Read the model definition and answer for the solid it produces. Units are mm, in the model's axes. Coordinates: 2 decimals unless noted, no trailing zeros. Order: outer loops, then holes, each group sorted by start corner. A loop starts at its lowest first (then second) coordinate and runs counter-clockwise, first axis right, second up. Notation, with made-up numbers: (61, 0.5) -> (67, 0.5) arc R25 ccw to (67, 24.5) -> close; hole circle Ø1 at (-13, 55). An arc over 180 degrees is marked (long way). Use CSV: the item, a comma, the result in double quotes.
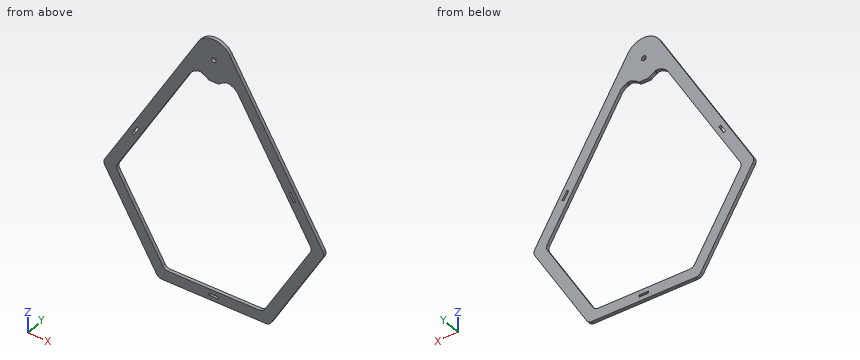
```python
from build123d import *

# Parameters (mm, degrees)
SKETCH1_R           = 4
BOSS_EXTRUDE1_DEPTH = 5.63
FILLET1_R           = 10
FILLET2_R           = 30
FILLET4_R           = 5


with BuildPart() as part:
    # Sketch1 → Boss-Extrude1 (new body)
    with BuildSketch(Plane(origin=(0, 0, 0), x_dir=(1, 0, 0), z_dir=(0, 1, 0))):
        Polygon((-36.68543943, -242.805029456), (146.099170261, 73.78720137), (54.706865415, 232.083316783), (-128.077744275, 232.083316783), (-219.470049121, 73.78720137), align=None)
        with Locations(Location((-36.68543943, -177.805029456, 0), (0, 0, 270))):
            Circle(SKETCH1_R, mode=Mode.SUBTRACT)
        with BuildLine():
            Line((67.466052068, -26.409354497), (3.019043242, -138.03484818))
            ThreePointArc((3.019043242, -138.03484818), (-2.040687786, -143.738783032), (-8.93543943, -146.994263122))
            Line((-8.93543943, -146.994263122), (-8.93543943, -148.494263122))
            Line((-8.93543943, -148.494263122), (-17.93543943, -148.494263122))
            Line((-17.93543943, -148.494263122), (-17.93543943, -146.994263122))
            ThreePointArc((-17.93543943, -146.994263122), (-23.578815596, -144.600710123), (-28.166359293, -140.53484818))
            Line((-28.166359293, -140.53484818), (-45.204519567, -140.53484818))
            ThreePointArc((-45.204519567, -140.53484818), (-49.792063264, -144.600710123), (-55.43543943, -146.994263122))
            Line((-55.43543943, -146.994263122), (-55.43543943, -148.494263122))
            Line((-55.43543943, -148.494263122), (-64.43543943, -148.494263122))
            Line((-64.43543943, -148.494263122), (-64.43543943, -146.994263122))
            ThreePointArc((-64.43543943, -146.994263122), (-71.330191074, -143.738783032), (-76.389922102, -138.03484818))
            Line((-76.389922102, -138.03484818), (-198.68543943, 73.78720137))
            Line((-198.68543943, 73.78720137), (-117.68543943, 214.083316783))
            Line((-117.68543943, 214.083316783), (44.31456057, 214.083316783))
            Line((44.31456057, 214.083316783), (125.31456057, 73.78720137))
            Line((125.31456057, 73.78720137), (67.466052068, -26.409354497))
        make_face(mode=Mode.SUBTRACT)
        Polygon((-44.534572815, 224.766675876), (-28.836306045, 224.99995769), (-28.836306045, 221.39995769), (-44.534572815, 221.39995769), align=None, mode=Mode.SUBTRACT)
        Polygon((-171.463513791, 5.037443083), (-168.345822337, 6.837443083), (-160.495822337, -6.759155756), (-163.613513791, -8.559155756), align=None, mode=Mode.SUBTRACT)
        Polygon((98.092634931, 5.037443083), (94.974943477, 6.837443083), (87.124943477, -6.759155756), (90.242634931, -8.559155756), align=None, mode=Mode.SUBTRACT)
    extrude(amount=BOSS_EXTRUDE1_DEPTH)

    # Fillet1
    fillet1_edges = [part.edges().sort_by_distance(p)[0] for p in [
        (125.31456057, 2.815, -73.78720137),
        (44.31456057, 2.815, -214.083316783),
        (-117.68543943, 2.815, -214.083316783),
        (-198.68543943, 2.815, -73.78720137),
        (146.099170261, 2.815, -73.78720137),
        (-219.470049121, 2.815, -73.78720137),
        (-128.077744275, 2.815, -232.083316783),
        (54.706865415, 2.815, -232.083316783),
    ]]
    fillet(fillet1_edges, radius=FILLET1_R)

    # Fillet2
    fillet2_edges = [part.edges().sort_by_distance(p)[0] for p in [
        (-36.68543943, 2.815, 242.805029456),
    ]]
    fillet(fillet2_edges, radius=FILLET2_R)

    # Fillet4
    fillet4_edges = [part.edges().sort_by_distance(p)[0] for p in [
        (-45.204519567, 2.815, 140.53484818),
        (-28.166359293, 2.815, 140.53484818),
    ]]
    fillet(fillet4_edges, radius=FILLET4_R)


solid = part.part
```
Item 1: Find section B-B, the plane z = -14.5. Give the vertices of the cut face in (x, y).
Return value:
outline,"(-185.24, 0) -> (-164.46, 0) -> (-164.46, 5.63) -> (-185.24, 5.63) -> close; (91.09, 0) -> (111.87, 0) -> (111.87, 5.63) -> (91.09, 5.63) -> close"
Item 2: Each of these flat-tipped pins is pushed along its axis until it touches: P1, Ø7, axis at x = -36.69, z = 177.81, coming from the -Y side; P2, Ø1.7, axis at y = 3, z = -223, coming from the +X side; P3, Ø2, axis at x = 98, y = 3.5, coming from the +Z side; P4, Ø1.6, axis at y = 3.5, z = 148, coming from the -X side. Where does it stop, or does it pass through?
Return value:
P1,"passes through"
P2,"stops at x = 60.44"
P3,"stops at z = 11.26"
P4,"stops at x = -91.88"
Item 3: Find section C-C, the plane y = 1.1. Give the number of separate pieces and of enclosed holes in the cut face, then the cut area to 3 significant figures.
Return value:
separate pieces,"1"
enclosed holes,"5"
area,"23,100 mm^2"
Item 4: Straight lines are drawn through the part: line 1 along X through (y, z) = (4.1, -42.5); line 2 along X through (y, z) = (2.9, -61); line 3 along Z through (x, y) = (22, 4.55). For each, find the intervals that lie inside material, in ascending order.
Return value:
line 1,"x = -201.41 to -180.62, 107.25 to 128.04"
line 2,"x = -212.09 to -191.3, 117.93 to 138.72"
line 3,"z = -232.08 to -214.08, 105.16 to 141.16"
Item 5: Find section A-A, the plane x = -97.5. Give the vertices of the cut face in (y, z).
Return value:
outline,"(0, -232.08) -> (5.63, -232.08) -> (5.63, -214.08) -> (0, -214.08) -> close; (0, 101.47) -> (5.63, 101.47) -> (5.63, 137.47) -> (0, 137.47) -> close"
